```python
from build123d import *

# Parameters (mm, degrees)
BASE_FLANGE1_DEPTH  = 2.5
SKETCH6_W           = 0.4
SKETCH6_H           = 3.67
BOSS_EXTRUDE1_DEPTH = 4.5
SKETCH8_W           = 3.4
SKETCH8_H           = 1
CUT_EXTRUDE1_DEPTH  = 4.5
FILLET1_RADIUS      = 1.335
FILLET1_LENGTH      = 0.4
FILLET2_R           = 0.05


# Sheet-metal steps are written as plain solids
with BuildPart() as part:
    # Sketch1 → Base-Flange1 (new body)
    with BuildSketch(Plane.XY):
        with BuildLine():
            Line((0.71, -1.835), (0.71, 1.835))
            ThreePointArc((0.71, 1.835), (0, 2.545), (-0.71, 1.835))
            Line((-0.71, 1.835), (-0.71, -1.835))
            Line((-0.71, -1.835), (-0.71, -2.335))
            ThreePointArc((-0.71, -2.335), (-1.228475759, -3.211432773), (-2.246268811, -3.179047252))
            Line((-2.246268811, -3.179047252), (-6.888528694, -0.229568793))
            Line((-6.888528694, -0.229568793), (-6.67402117, 0.108050107))
            Line((-6.67402117, 0.108050107), (-2.031761286, -2.841428351))
            ThreePointArc((-2.031761286, -2.841428351), (-1.421085455, -2.860859664), (-1.11, -2.335))
            Line((-1.11, -2.335), (-1.11, -1.835))
            Line((-1.11, -1.835), (-1.11, 1.835))
            ThreePointArc((-1.11, 1.835), (0, 2.945), (1.11, 1.835))
            Line((1.11, 1.835), (1.11, -1.835))
            Line((1.11, -1.835), (0.71, -1.835))
        make_face()
    extrude(amount=BASE_FLANGE1_DEPTH)

    # Sketch6 → Boss-Extrude1 (add)
    with BuildSketch(Plane.XY.offset(2.5)):
        with Locations((0.91, 0)):
            Rectangle(SKETCH6_W, SKETCH6_H)
    extrude(amount=BOSS_EXTRUDE1_DEPTH)

    # Sketch8 → Cut-Extrude1 (cut)
    with BuildSketch(Plane(origin=(1.11, 0, 0), x_dir=(0, 0, -1), z_dir=(1, 0, 0))):
        with Locations((-5.3, -1.335)):
            Rectangle(SKETCH8_W, SKETCH8_H)
    extrude(amount=-CUT_EXTRUDE1_DEPTH, mode=Mode.SUBTRACT)

    # Fillet1: full round fillet: the end face becomes a half cylinder, R = half its width
    fillet1_face = Plane((0.91, 0.5, 7), x_dir=(-1, 0, 0), z_dir=(0, 0, 1))  # on the end face: x along it, z out of the body
    fillet1_slab = fillet1_face.offset(-FILLET1_RADIUS / 2) * Box(FILLET1_LENGTH, 2 * FILLET1_RADIUS, FILLET1_RADIUS, mode=Mode.PRIVATE)  # the body's end, R deep
    fillet1_round = Plane((0.91, 0.5, 5.665), x_dir=(0, 0, 1), z_dir=(-1, 0, 0)) * Cylinder(FILLET1_RADIUS, FILLET1_LENGTH, mode=Mode.PRIVATE)  # its axis R under the face
    add(fillet1_slab - fillet1_round, mode=Mode.SUBTRACT)

    # Fillet2
    fillet2_edges = [part.edges().sort_by_distance(p)[0] for p in [
        (1.11, -0.835, 4.6325),
        (0.71, 1.835, 4.0825),
        (1.11, 1.835, 4.0825),
        (0.71, -0.835, 4.6325),
        (0.71, 0.5, 7),
        (1.11, 0.5, 7),
    ]]
    fillet(fillet2_edges, radius=FILLET2_R)


solid = part.part
```
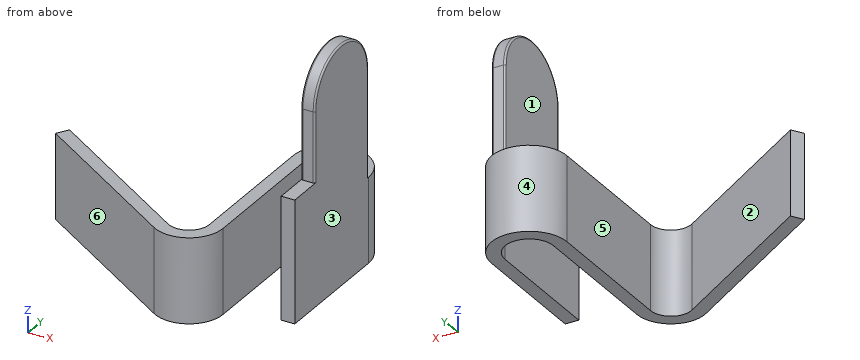
CAD build for the part. Positions are in the model's coordinates, mm. Face numbers are marked on the shaded views. A direction names the side the tool comes from. Round coordinates to 2 decimals unless told otherwise and drop trailing zeros. Order: outer loops, then holes, each group sorted by start corner. A loop starts at its lowest first (then second) coordinate and runs counter-clockwise, first axis right, second up.
Q1. Drop flat-ended pins along their axis: pin 1 (3 mm diameter, centred on x = -3.5, z = 1, fed in from -Y); pin 2 (1 mm diameter, centred on y = -1.5, z = 2, fed in from -X); pin 3 (2 mm diameter, centred on x = -4, z = 4.5, fed in from -Y); pin 4 (3 mm diameter, centred on x = -4, y = 0, fed in from +Z). Give the stop position or say it passes through.
Q2. Which spindle directions (+Z, -Z, +X, -X, +Y, -Y) get a long thin tool onto all of the face, cutting with end or side? Do the marked faces 1 and 2. Say none if no direction does.
Q3. Slice it at A-A (y = 0.5). Write the cut outline in (x, z), and give its area (3 significant figures).
Q4. Wall check: L1, parallel to X at y = 0, z = 4; L2, parallel to X at y = 1.75, z = 0.75; L3, parallel to Z at x = -1, y = 2. Give the ranges that are in metal, low to high.
Q5. Slice it at D-D (z = 2.75). Write the cut outline in (x, y) (3 decimals), and give its area (3 significant figures).
Q6. Two-plate mould, pull along X, no slides. Class the marked faces 3, 4, 5 and 6: pulls with the +X half, pulls with the -X half, needs draft (parallel to the pull), parting line crosses it, or undercut.
Q7. Slice it at C-C (x = 0). Write the cut outline in (y, z) (3 decimals), and give its area (4 significant figures).
Q8. Slice it at B-B (z = 1). Write the cut outline in (x, y) (3 decimals).
Results below:
1. pin 1: stops at y = -3.29
1. pin 2: stops at x = -5.68
1. pin 3: passes through
1. pin 4: stops at z = 2.5
2. face 1: +Z, -Z, -Y
2. face 2: +Z, -Z, +Y
3. outline: (-1.11, 0) - (-0.71, 0) - (-0.71, 2.5) - (-1.11, 2.5) - close; (0.71, 0) - (1.11, 0) - (1.11, 6.95) arc R0.05 ccw to (1.06, 7) - (0.76, 7) arc R0.05 ccw to (0.71, 6.95) - close
3. area: 3.80 mm2
4. L1: x = 0.71 to 1.11
4. L2: x = -1.11 to -0.71, 0.71 to 1.11
4. L3: z = 0 to 2.5
5. outline: (0.71, -1.835) - (1.11, -1.835) - (1.11, 1.785) arc R0.05 ccw to (1.06, 1.835) - (0.76, 1.835) arc R0.05 ccw to (0.71, 1.785) - close
5. area: 1.47 mm2
6. face 3: pulls with the +X half
6. face 4: parting line crosses it
6. face 5: undercut
6. face 6: pulls with the -X half
7. outline: (2.545, 0) - (2.945, 0) - (2.945, 2.5) - (2.545, 2.5) - close
7. area: 1.000 mm2
8. outline: (-6.889, -0.23) - (-2.246, -3.179) arc R1 ccw to (-0.71, -2.335) - (-0.71, 1.835) arc R0.71 cw to (0.71, 1.835) - (0.71, -1.835) - (1.11, -1.835) - (1.11, 1.835) arc R1.11 ccw to (-1.11, 1.835) - (-1.11, -2.335) arc R0.6 cw to (-2.032, -2.841) - (-6.674, 0.108) - close
